Input: part model. Units: mm. Frame: model coordinates. A direction names the side the tool comes from. Round coordinates to 2 decimals unless told otherwise and drop trailing zeros. Loops run counter-clockwise (first coordinate to the right, second up) from the corner with the lowest first, then second, coordinate; pieces in that order, holes last. Notation, with made-up numbers: M 16,56 L 39,56 A24 cw 39,89 Z; hole C -7,63 d2. An arc over 180 degrees is marked long. Use one line per item in the form item = value. Start each with the question number.
Q1. Section query A-A, the plane x = -12. Output: boundary loops of the cut face in (y, z).
Q2. Ray query, line 1 along Z through (x, y) = (-16, 17.5); line 2 along X through (y, z) = (12.5, -22.5); line 3 along Z through (x, y) = (-31.5, 20). Return the intervals inside material, ascending.
Q3. Section query B-B, the plane z = 22.5. Output: boundary loops of the cut face in (x, y).
Q4. First-contact query: P1, Ø7, axis at x = -31.5, z = -17.5, coming from the +Y side; P2, Ø5, axis at x = 40.02, z = 10.81, coming from the +Y side; P3, Ø2, axis at x = 40, z = -19.5, coming from the +Y side; P4, Ø1.5, axis at y = 20, z = -34.19, coming from the -X side. Flat tips, straight axial feed; report the tip coordinate or a pass-through.
Q5. Mould query, pull axis Y, two halves, no side actions, for faces 6 (the flat face through (-32, 3, 12)), 7 (the cylindrical face through (-31.176, 20.479, 26.967)), 8 (the flat face through (-31, 30, -29.188)). Classes: pulls with the +Y half, pulls with the -Y half, needs draft (parallel to the pull), parting line crosses it, or undercut.
Q6. Section query C-C, the plane y = 4.5. Output: boundary loops of the cut face in (x, z), and give its area (3 significant figures).
Q7. Section query D-D, the plane z = -19.5. Output: boundary loops of the cut face in (x, y).
Q8. Access query for faces 1 (the flat face through (40, 25, -5)), 2 (the flat face through (4, 25, -37)), 3 (the flat face through (4, 13, 26.312)), 4 (the flat face through (-31, 15, 7)), 5 (the flat face through (38.6, 3, 12.2)). Directions: +Z, -Z, +X, -X, +Y, -Y. A direction counts if a zero-diameter tool reaches every point of the face in a straight line with its end or side. Return the directions, or none.
```python
from build123d import *

# Parameters (mm, degrees)
SKETCH1_W                       = 80
SKETCH1_H                       = 70
BOSS_EXTRUDE1_DEPTH             = 25
SKETCH2_W                       = 61
SKETCH2_H                       = 61
CUT_EXTRUDE1_DEPTH              = 26
SKETCH3_W                       = 9.5
SKETCH3_H                       = 10
BOSS_EXTRUDE2_DEPTH             = 10
FILLET1_R                       = 2
FILLET4_R                       = 2
CBORE_FOR_M3_SHCS1_D            = 3.4
CBORE_FOR_M3_SHCS1_CBORE_D      = 6.5
CBORE_FOR_M3_SHCS1_CBORE_DEPTH  = 22
TAP_DRILL_FOR_M3X0_5_TAP1_D     = 2.5
TAP_DRILL_FOR_M3X0_5_TAP1_DEPTH = 8
TAP_DRILL_FOR_M3X0_5_TAP1_TIP   = 0.751075774
CUT_EXTRUDE2_REACH              = 82
SKETCH9_W                       = 20
SKETCH9_H                       = 10
FILLET5_R                       = 2


with BuildPart() as part:
    # Sketch1 → Boss-Extrude1 (new body)
    with BuildSketch(Plane(origin=(0, 0, 0), x_dir=(1, 0, 0), z_dir=(0, 1, 0))):
        with Locations((4.767506632, 4.187819453)):
            Rectangle(SKETCH1_W, SKETCH1_H)
    extrude(amount=BOSS_EXTRUDE1_DEPTH)

    # Sketch2 → Cut-Extrude1 (cut, through all)
    with BuildSketch(Plane(origin=(0, 25, 0), x_dir=(1, 0, 0), z_dir=(0, 1, 0))):
        with Locations((4.767506632, 4.187819453)):
            Rectangle(SKETCH2_W, SKETCH2_H)
    extrude(amount=-CUT_EXTRUDE1_DEPTH, mode=Mode.SUBTRACT)

    # Sketch3 → Boss-Extrude2 (add)
    with BuildSketch(Plane(origin=(0, 25, 0), x_dir=(1, 0, 0), z_dir=(0, 1, 0))):
        with Locations((-30.482493368, 34.187819453)):
            Rectangle(SKETCH3_W, SKETCH3_H)
        with Locations((40.017506632, 34.187819453)):
            Rectangle(SKETCH3_W, SKETCH3_H)
        with Locations((-30.482493368, -25.812180547)):
            Rectangle(SKETCH3_W, SKETCH3_H)
        with Locations((40.017506632, -25.812180547)):
            Rectangle(SKETCH3_W, SKETCH3_H)
    extrude(amount=BOSS_EXTRUDE2_DEPTH)

    # Fillet1
    fillet1_edges = [part.edges().sort_by_distance(p)[0] for p in [
        (44.767506632, 17.5, 30.812180547),
    ]]
    fillet(fillet1_edges, radius=FILLET1_R)

    # Fillet4
    fillet4_edges = [part.edges().sort_by_distance(p)[0] for p in [
        (44.767506632, 17.5, -39.187819453),
    ]]
    fillet(fillet4_edges, radius=FILLET4_R)

    # CBORE for M3 SHCS1 (through all)
    with Locations(Plane(origin=(-30.482493368, 25, -19.187819453), x_dir=(0, 0, 1), z_dir=(0, 1, 0))):
        with Locations((0, 0), (30, 0), (30, 70.5), (0, 70.5)):
            CounterBoreHole(CBORE_FOR_M3_SHCS1_D / 2, CBORE_FOR_M3_SHCS1_CBORE_D / 2, CBORE_FOR_M3_SHCS1_CBORE_DEPTH)

    # Tap Drill for M3x0.5 Tap1
    with Locations(Plane(origin=(-35.232493368, 20, 25.812180547), x_dir=(0, 0, -1), z_dir=(-1, 0, 0))):
        with Locations((0, 0), (60, 0)):
            Hole(TAP_DRILL_FOR_M3X0_5_TAP1_D / 2, depth=TAP_DRILL_FOR_M3X0_5_TAP1_DEPTH)
            with Locations((0, 0, -(TAP_DRILL_FOR_M3X0_5_TAP1_DEPTH + TAP_DRILL_FOR_M3X0_5_TAP1_TIP / 2))):  # 118° drill point
                Cone(0, TAP_DRILL_FOR_M3X0_5_TAP1_D / 2, TAP_DRILL_FOR_M3X0_5_TAP1_TIP, mode=Mode.SUBTRACT)

    # Sketch9 → Cut-Extrude2 (cut, up to next)
    with BuildSketch(Plane.ZY.offset(35.232493368), mode=Mode.PRIVATE) as cut_extrude2_sk1:
        with Locations((10.812180547, 20)):
            Rectangle(SKETCH9_W, SKETCH9_H)
    cut_extrude2_tool1 = extrude(cut_extrude2_sk1.sketch, amount=-CUT_EXTRUDE2_REACH, mode=Mode.PRIVATE) & part.part
    add(cut_extrude2_tool1.solids().sort_by_distance((-35.232493, 20, 10.812181))[0], mode=Mode.SUBTRACT)

    # Fillet5
    fillet5_edges = [part.edges().sort_by_distance(p)[0] for p in [
        (-30.482493368, 15, 0.812180547),
        (-30.482493368, 15, 20.812180547),
    ]]
    fillet(fillet5_edges, radius=FILLET5_R)


solid = part.part
```
Results found:
q1.outline = M 0,-39.19 L 25,-39.19 L 25,-34.69 L 0,-34.69 Z; M 0,26.31 L 25,26.31 L 25,30.81 L 0,30.81 Z
q2.line_1 = -39.19 to -34.69, 26.31 to 30.81
q2.line_2 = -35.23 to -25.73, 35.27 to 44.77
q2.line_3 = -39.19 to -35.44, -32.94 to -22.27, -16.1 to 0.81, 20.81 to 24.56, 27.06 to 30.81
q3.outline = M -35.23,0 L -25.73,0 L -25.73,35 L -35.23,35 Z; M 35.27,0 L 44.77,0 L 44.77,35 L 35.27,35 Z
q4.P1 = 25
q4.P2 = 3
q4.P3 = through
q4.P4 = -26.93
q5.face_6 = pulls with the +Y half
q5.face_7 = undercut
q5.face_8 = needs draft
q6.outline = M -35.23,-39.19 L 42.77,-39.19 A2 ccw 44.77,-37.19 L 44.77,28.81 A2 ccw 42.77,30.81 L -35.23,30.81 Z; hole C -30.48,-19.19 d6.5; hole C -30.48,10.81 d6.5; hole M -25.73,-34.69 L 35.27,-34.69 L 35.27,26.31 L -25.73,26.31 Z; hole C 40.02,-19.19 d6.5; hole C 40.02,10.81 d6.5
q6.area = 1,740 mm²
q7.outline = M -35.23,0 L -32.15,0 L -32.15,3 L -33.72,3 L -33.72,25 L -35.23,25 Z; M -28.81,0 L -25.73,0 L -25.73,25 L -27.25,25 L -27.25,3 L -28.81,3 Z; M 35.27,0 L 38.35,0 L 38.35,3 L 36.78,3 L 36.78,25 L 35.27,25 Z; M 41.69,0 L 44.77,0 L 44.77,25 L 43.25,25 L 43.25,3 L 41.69,3 Z
q8.face_1 = +X, -X, +Y
q8.face_2 = +Z, -Z, +Y
q8.face_3 = +Y, -Y
q8.face_4 = -X, +Y
q8.face_5 = +Y
